Geometry check sheet. Reference: drawing and pictorial views, mm from the part's lowest x, y, z. A direction names the side the tool comes from. Coordinates: 2 decimals unless noted, no trailing zeros. Order: outer loops, then holes, each group sorted by start corner. A loop starts at its lowest first (then second) coordinate and runs counter-clockwise, first axis right, second up. Notation, with made-up numbers: (21.5, -29) -> (60.5, -29) arc R24 cw to (60.5, -4) -> close; hole circle Ø6 at (-12.75, 56). An arc over 180 degrees is marked (long way). Use CSV: the item, a comma, the result in double quotes. Start each with the question number.
1) Release check for a two-part mould opening along Y. For the marked faces 3, 4 and 5 record: released by +Y, released by -Y, zero draft, split by the parting line, or undercut.
2) Sectioned sample at C-C on z = 4.05. Record the boundary of the cut face in (x, y), then the cut area to 3 significant figures.
3) Tool access check on the marked faces 1 and 2. Record the directions out of +Z, -Z, +X, -X, +Y, -Y that give a thin tool (end or side, any length) a straight path to the whole face; none if there is none.
4) Scan lines: line 1 along Y through (x, z) = (7, 1.4); line 2 along Z through (x, y) = (8.25, 5); line 3 along X through (y, z) = (7.25, 2.3). Record each from-to range of solid material in increasing order.
5) Go/stop test with flat-tipped pins: pin 1 (1.5 mm diameter, centred on y = 6, z = 2.5, fed in from +X); pin 2 (2 mm diameter, centred on x = 2, y = 7.5, fed in from -Z). Record where each tip stops, or that it passes through.
6) Sectioned sample at B-B on z = 1. Record the boundary of the cut face in (x, y), then the cut area to 3 significant figures.
7) Sectioned sample at A-A on x = 7. Record the boundary of the cut face in (y, z), then the cut area to 3 significant figures.
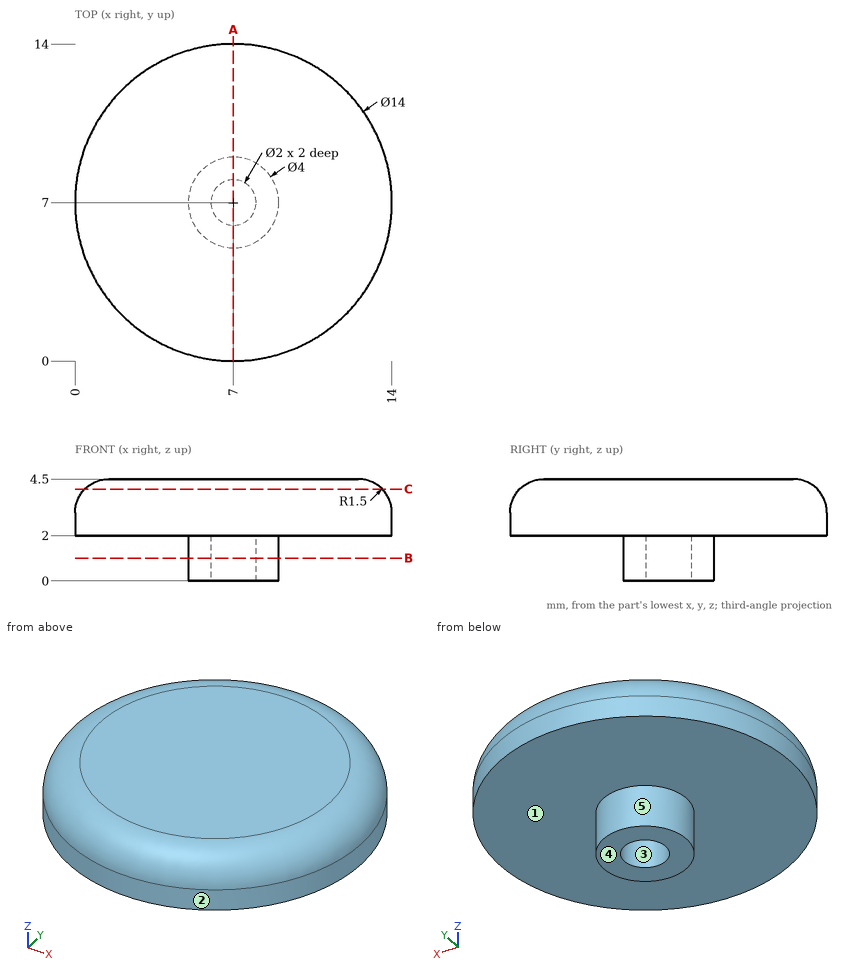
Answers follow:
1,face 3,"undercut"
1,face 4,"zero draft"
1,face 5,"split by the parting line"
2,outline,"circle Ø13.14 at (7, 7)"
2,area,"136 mm²"
3,face 1,"-Z"
3,face 2,"+Z, -Z"
4,line 1,"y = 5 to 6, 8 to 9"
4,line 2,"z = 2 to 4.5"
4,line 3,"x = 0 to 14"
5,pin 1,"stops at x = 14"
5,pin 2,"stops at z = 2"
6,outline,"circle Ø4 at (7, 7); hole circle Ø2 at (7, 7)"
6,area,"9.42 mm²"
7,outline,"(0, 2) -> (5, 2) -> (5, 0) -> (6, 0) -> (6, 2) -> (8, 2) -> (8, 0) -> (9, 0) -> (9, 2) -> (14, 2) -> (14, 3) arc R1.5 ccw to (12.5, 4.5) -> (1.5, 4.5) arc R1.5 ccw to (0, 3) -> close"
7,area,"38.0 mm²"
